The listing builds one solid part. Answer for the finished solid, in the listing's coordinates (mm). A direction names the side the tool comes from. Coordinates: 2 decimals unless noted, no trailing zeros. Loops run counter-clockwise (first coordinate to the right, second up) from the corner with the lowest first, then second, coordinate; pieces in that order, holes last. Notation, with made-up numbers: (33.5, 53.5) - (77.5, 53.5) arc R10 ccw to (77.5, 57.5) - close; hole circle Ø3 at (49, -8). An arc over 180 degrees is marked (long way). Put each result on its own line as item: value.
```python
from build123d import *

# Parameters (mm, degrees)
F1_DEPTH = 30
F2_R     = 2.75
F3_DEPTH = 3.5
F4_R     = 5
F5_DEPTH = 16.7248737342
F6_R     = 1.6
F7_DEPTH = 3.5
F8_DEPTH = 2


with BuildPart() as f1:
    # F0 (on Front) → F1 (new body)
    with BuildSketch(Plane.XZ):
        Polygon((0, 3.5), (0, 0), (20, 0), (20, 3.5), (4.2248737342, 3.5), align=None)
        with BuildLine():
            ThreePointArc((1.75, 5.9748737342), (0.7696146381, 4.8119555711), (0, 3.5))
            Line((0, 3.5), (4.2248737342, 3.5))
            Line((4.2248737342, 3.5), (1.75, 5.9748737342))
        make_face()
        Polygon((1.75, 5.9748737342), (4.2248737342, 3.5), (21.7124208231, 20.987547089), (19.237547089, 23.4624208231), align=None)
    extrude(amount=F1_DEPTH)

    # F2 (on face) → F3 (cut, through all)
    with BuildSketch(Plane(origin=(0, 0, 0), x_dir=(1, 0, 0), z_dir=(0, 0, -1))):
        with Locations((10, 15)):
            Circle(F2_R)
    extrude(amount=-F3_DEPTH, mode=Mode.SUBTRACT)

    # F4 (on face) → F5 (cut, up to face)
    with BuildSketch(Plane.XY.offset(3.5)):
        with Locations((10, -15)):
            Circle(F4_R)
    extrude(amount=F5_DEPTH, mode=Mode.SUBTRACT)

    # F6 (on face) → F7 (cut, through all)
    with BuildSketch(Plane(origin=(0.3624368671, 0, -0.3624368671), x_dir=(0, 1, 0), z_dir=(0.7071067812, 0, -0.7071067812))):
        with Locations((-5.221, 17.8278737342)):
            Circle(F6_R)
        with Locations((-24.779, 17.8278737342)):
            Circle(F6_R)
    extrude(amount=-F7_DEPTH, mode=Mode.SUBTRACT)

    # F6 (on face) → F8 (cut)
    with BuildSketch(Plane(origin=(0.3624368671, 0, -0.3624368671), x_dir=(0, 1, 0), z_dir=(0.7071067812, 0, -0.7071067812))):
        Polygon((-21.879, 19.5021895148), (-24.779, 21.1765052955), (-27.679, 19.5021895148), (-27.679, 16.1535579535), (-24.779, 14.4792421729), (-21.879, 16.1535579535), align=None)
        with Locations((-24.779, 17.8278737342)):
            Circle(F6_R, mode=Mode.SUBTRACT)
        Polygon((-8.121, 16.1535579535), (-5.221, 14.4792421729), (-2.321, 16.1535579535), (-2.321, 19.5021895148), (-5.221, 21.1765052955), (-8.121, 19.5021895148), align=None)
        with Locations((-5.221, 17.8278737342)):
            Circle(F6_R, mode=Mode.SUBTRACT)
    extrude(amount=-F8_DEPTH, mode=Mode.SUBTRACT)


solid = f1.part
```
1) The part is cut by section D-D (x = 10). State how many separate pieces and enclosed holes the cut face has, and give its area (3 significant figures).
Found:
separate pieces: 4
enclosed holes: 2
area: 173 mm^2
2) For faces 1 (the face through (11.5, -10.23, 12.17)), 2 (the face through (20, -15, 2)), 3 (the face through (14, -15, 3.5)), 4 (the face through (10.487, -23.349, 11.157)), 5 (the face through (10.535, -23.531, 12.639)), determine the directions among +Z, -Z, +X, -X, +Y, -Y from which every point of the face is accessible in a straight line to the end or side of a thin tool.
Found:
face 1: +Z
face 2: -Z, +X, +Y, -Y
face 3: +X, +Y, -Y
face 4: +X
face 5: none
3) The part is cut by section B-B (x = 18.5). Give the vertices of the cut face in (y, z).
Found:
outline: (-30, 0) - (0, 0) - (0, 3.5) - (-30, 3.5) - close; (-30, 17.78) - (0, 17.78) - (0, 22.72) - (-30, 22.72) - close
4) The part is cut by section C-C (z = 2.75). Give the vertices of the cut face in (x, y), and give its area (3 significant figures).
Found:
outline: (0, -30) - (20, -30) - (20, 0) - (0, 0) - close; hole circle Ø5.5 at (10, -15)
area: 576 mm^2
5) Each of these flat-tipped pins is pushed along its axis until it touches: pin 1 (1 mm diameter, centred on y = -13.5, z = 1.5, fed in from +X); pin 2 (4.5 mm diameter, centred on x = 10, y = -15, fed in from +Z); pin 3 (2 mm diameter, centred on x = 16.5, y = -16, fed in from +Z); pin 4 (12.5 mm diameter, centred on x = 12.5, y = -11, fed in from +Z). Where does it stop, or does it pass through?
Found:
pin 1: stops at x = 20
pin 2: passes through
pin 3: stops at z = 21.72
pin 4: stops at z = 22.97
6) The part is cut by section A-A (y = -15). Give the vertices of the cut face in (x, z).
Found:
outline: (0, 0) - (7.25, 0) - (7.25, 3.5) - (4.22, 3.5) - (5, 4.28) - (5, 9.22) - (1.75, 5.97) arc R8.96 ccw to (0, 3.5) - close; (12.75, 0) - (20, 0) - (20, 3.5) - (12.75, 3.5) - close; (15, 14.28) - (21.71, 20.99) - (19.24, 23.46) - (15, 19.22) - close
7) For a pull along Z with two mould halves and no side action, classify faces 6 (the face through (10.535, -6.55, 12.639)), 7 (the face through (9, 0, 9)), 8 (the face through (10, -11, 0)), 9 (the face through (0.78, -14.79, 4.83)) as pulls with the +Z half, pulls with the -Z half, needs draft (parallel to the pull), parting line crosses it, or undercut.
Found:
face 6: undercut
face 7: needs draft
face 8: pulls with the -Z half
face 9: pulls with the +Z half
8) Straight lines are drawn through the part: L1, parallel to Y at x = 10, z = 0.7; L2, parallel to X at y = -15, z = 2.2; L3, parallel to Z at x = 13.5, y = -25. For each, find the intervals that lie inside material, in ascending order. Write a range as [from, to].
Found:
L1: y = [-30, -17.75], [-12.25, 0]
L2: x = [0, 7.25], [12.75, 20]
L3: z = [0, 3.5], [15.6, 17.72]
